Autodesk Inventor part; units mm, degrees
ref_plane "YZ Plane" through (0, 0, 0) normal (1, 0, 0) x (0, 1, 0)
ref_plane "XZ Plane" through (0, 0, 0) normal (0, 1, 0) x (-1, 0, 0)
ref_plane "XY Plane" through (0, 0, 0) normal (0, 0, 1) x (1, 0, 0)
sketch "Sketch2" plane through (0, 0, 0) normal (0, 0, 1) x (1, 0, 0)
  line L0 (0, 0) -> (19.05, 0)
  line L1 (19.05, 0) -> (19.05, 19.05)
  line L2 (19.05, 19.05) -> (15.875, 19.05) construction
  line L3 (15.875, 19.05) -> (15.875, 22.225) construction
  line L4 (15.875, 22.225) -> (19.05, 19.05)
  line L5 (15.875, 22.225) -> (0, 22.225)
  line L6 (0, 22.225) -> (0, 0)
  dimension "d3" = 19.05
  dimension "d4" = 19.05
  dimension "d10" = 3.175
  dimension "d11" = 3.175
revolve "Revolution2" add sketch "Sketch2" angle 360 about axis through (0, 22.225, 0) along (0, -1, 0)
sketch "Sketch4" plane through (0, 22.225, 0) normal (0, 1, 0) x (1, 0, 0)
  circle A0 centre (0, 0) radius 15.875
extrude "Extrusion3" cut sketch "Sketch4" against normal blind 12.7
sketch "Sketch6" plane through (0, 0, 0) normal (0, -1, 0) x (1, 0, 0)
  circle A0 centre (0, 0) radius 15.875
  circle A1 centre (0, 0) radius 13.97
  circle A2 centre (0, 0) radius 19.05
  dimension "d48" = 27.94
extrude "Extrusion5" cut sketch "Sketch6" against normal blind 1.25
properties part number "base_1.0"
The listing builds one solid part. Answer for the finished solid, in the listing's coordinates (mm). A direction names the side the tool comes from. Give positions to 0.01 mm unless a question says otherwise; leave off trailing zeros. Order: outer loops, then holes, each group sorted by start corner. A loop starts at its lowest first (then second) coordinate and runs counter-clockwise, first axis right, second up.
Item 1: The part is cut by section A-A, the plane z = 0. Give the vertices of the cut face in (x, y) (3 decimals), and give its area (3 significant figures).
From the geometry:
outline: (-19.05, 1.25) - (-15.875, 1.25) - (-15.875, 0) - (-13.97, 0) - (-13.97, 1.25) - (13.97, 1.25) - (13.97, 0) - (15.875, 0) - (15.875, 1.25) - (19.05, 1.25) - (19.05, 19.05) - (15.875, 22.225) - (15.875, 9.525) - (-15.875, 9.525) - (-15.875, 22.225) - (-19.05, 19.05) - close
area: 391 mm2
Item 2: The part is cut by section D-D, the plane y = 17.25. Give the vertices of the cut face in (x, z) (3 decimals), and give its area (3 significant figures).
From the geometry:
outline: circle Ø38.1 at (0, 0); hole circle Ø31.75 at (0, 0)
area: 348 mm2
Item 3: For a pull along X with two mould halves and no side action, classify faces 1 (the face through (0, 9.525, 0)), 2 (the face through (-15.12, 10.27, 11.59)), 3 (the face through (0, 1.25, 0)), 4 (the face through (9, 0, -11)) as pulls with the +X half, pulls with the -X half, needs draft (parallel to the pull), parting line crosses it, or undercut.
From the geometry:
face 1: undercut
face 2: parting line crosses it
face 3: undercut
face 4: needs draft
Item 4: The part is cut by section C-C, the plane y = 6.75. Give the vertices of the cut face in (x, z).
From the geometry:
outline: circle Ø38.1 at (0, 0)
Item 5: Find the intervals of material crossed by probe 1 along Z at (x, y) = (0, 0.3) (3 decimals); probe 2 along Z at (x, y) = (-0.5, 12.5); probe 3 along Y at (x, z) = (-5, -9) (3 decimals), in increasing order.
From the geometry:
probe 1: z = -15.875 to -13.97, 13.97 to 15.875
probe 2: z = -19.04 to -15.87, 15.87 to 19.04
probe 3: y = 1.25 to 9.525
Item 6: Which of the six approach directions +Z, -Z, +X, -X, +Y, -Y give full straight-line access (tool end or side, diameter ignored) to faces 5 (the face through (-4, 1.25, 16)), 6 (the face through (-3.441, 15.964, 15.497))?
From the geometry:
face 5: -Y
face 6: +Y
Item 7: The part is cut by section B-B, the plane x = 0. Give the vertices of the cut face in (y, z) (3 decimals), and give its area (3 significant figures).
From the geometry:
outline: (0, -15.875) - (1.25, -15.875) - (1.25, -19.05) - (19.05, -19.05) - (22.225, -15.875) - (9.525, -15.875) - (9.525, 15.875) - (22.225, 15.875) - (19.05, 19.05) - (1.25, 19.05) - (1.25, 15.875) - (0, 15.875) - (0, 13.97) - (1.25, 13.97) - (1.25, -13.97) - (0, -13.97) - close
area: 391 mm2
Item 8: Given pin 1 Ø12 at (x, z) = (5, -1) entering from +Y (3 decimals); pin 2 Ø22.5 at (x, z) = (0, 0) entering from -Y; pin 3 Ø3 at (x, y) = (-12.5, 11) entering from +Z, each flat-ended and moving along its own axis, determine where each tip first touches the part or whether it passes through.
From the geometry:
pin 1: stops at y = 9.525
pin 2: stops at y = 1.25
pin 3: stops at z = 15.55
